from build123d import *

# Parameters (mm, degrees)
BOSS_EXTRUDE1_DEPTH = 2
BOSS_EXTRUDE2_DEPTH = 8


with BuildPart() as part:
    # Sketch1 → Boss-Extrude1 (new body)
    with BuildSketch(Plane(origin=(0, 0, 0), x_dir=(1, 0, 0), z_dir=(0, 1, 0))):
        Polygon((0, 0), (32, 0), (32, -6), (6, -6), (6, -32), (0, -32), align=None)
    extrude(amount=BOSS_EXTRUDE1_DEPTH)

    # Sketch2 → Boss-Extrude2 (add)
    with BuildSketch(Plane(origin=(0, 2, 0), x_dir=(1, 0, 0), z_dir=(0, 1, 0))):
        Polygon((2, -32), (2, -2), (32, -2), (32, 0), (0, 0), (0, -32), align=None)
        Polygon((32, -4.1), (4.1, -4.1), (4.1, -32), (6, -32), (6, -6), (32, -6), align=None)
    extrude(amount=BOSS_EXTRUDE2_DEPTH)


solid = part.part
Source: CAD feature listing. Evaluate the final solid. Frame: model axes, mm. A direction names the side the tool comes from. Give positions to 0.01 mm unless a question says otherwise; leave off trailing zeros. Write each loop counter-clockwise with the first axis right and the second up, starting at its lowest first coordinate (ties: lowest second). Pieces come first, ordered by that corner, then holes. Notation, with made-up numbers: M 77,79 L 81,79 A21 cw 81,90 Z; hole C 82,-10.5 d1. An arc over 180 degrees is marked long. Return JSON: item names as keys, results as strings. Group by question number.
1) Cut plane A-A, the plane y = 7.75. Output: boundary loops of the cut face in (x, z), then the cut area to 3 significant figures.
2) First-contact query: pin 1 Ø5 at (x, z) = (7, 4.5) entering from -Y; pin 2 Ø3 at (y, z) = (7.5, 21.5) entering from +X; pin 3 Ø4 at (x, y) = (17.5, 6.5) entering from +Z; pin 4 Ø8 at (x, z) = (21.5, 13.5) entering from -Y. Flat tips, straight axial feed; report the tip coordinate or a pass-through.
3) Draft query along Z for faces 1 (the face through (17, 6, 2)), 2 (the face through (1.6, 4.9, 32)), 3 (the face through (32, 4.9, 4.4)). Return one class per face: released by +Z, released by -Z, zero draft, split by the parting line, or undercut.
4) Set-up query: faces 4 (the face through (0, 5, 16)), 5 (the face through (19, 5, 6)), 6 (the face through (18, 6, 4.1)), 7 (the face through (1.7, 10, 8.8)), 8 (the face through (4.1, 6, 18)). Return all of +Z, -Z, +X, -X, +Y, -Y with unobstructed straight access to the full face (end or side cutting, diameter ignored); none if empty.
5) Cut plane B-B, the plane x = 25. Output: boundary loops of the cut face in (y, z), then the cut area to 3 significant figures.
6) Ray query, L1, parallel to X at y = 5, z = 7; L2, parallel to Z at x = 2.5, y = 4. Return the intervals inside material, ascending.
7) Cut plane C-C, the plane z = 4.5. Output: boundary loops of the cut face in (x, y), then the cut area to 3 significant figures.
Data:
{
 "1": {"outline": "M 0,0 L 32,0 L 32,2 L 2,2 L 2,32 L 0,32 Z; M 4.1,4.1 L 32,4.1 L 32,6 L 6,6 L 6,32 L 4.1,32 Z", "area": "226 mm²"},
 "2": {"pin 1": "stops at y = 0", "pin 2": "stops at x = 6", "pin 3": "stops at z = 6", "pin 4": "passes through"},
 "3": {"face 1": "undercut", "face 2": "released by +Z", "face 3": "zero draft"},
 "4": {"face 4": "+Z, -Z, -X, +Y, -Y", "face 5": "+Z, +X, +Y, -Y", "face 6": "+X, +Y", "face 7": "+Z, -Z, +X, -X, +Y", "face 8": "+Z, +Y"},
 "5": {"outline": "M 0,0 L 10,0 L 10,2 L 2,2 L 2,4.1 L 10,4.1 L 10,6 L 0,6 Z", "area": "43.2 mm²"},
 "6": {"L1": "x = 0 to 2, 4.1 to 6", "L2": "z = 0 to 2"},
 "7": {"outline": "M 0,0 L 32,0 L 32,10 L 4.1,10 L 4.1,2 L 2,2 L 2,10 L 0,10 Z", "area": "303 mm²"}
}
